```python
from build123d import *

# Parameters (mm, degrees)
F0_R          = 7.6724970278
F1_DEPTH      = 25.4
F1_TAPER      = 3
F1_DEPTH_BACK = 25.4
F1_TAPER_BACK = 3
F4_DEPTH      = 25.4
F4_TAPER      = 3
F4_DEPTH_BACK = 13.716
F6_W          = 8.5597652942
F6_H          = 9.2730754986
F7_DEPTH      = 4.572
F8_R          = 1.5035458926
F9_DEPTH      = 6.5786
F10_R         = 4.568572737
F11_DEPTH     = 53.594


with BuildPart() as f1:
    # F0 (on Front) → F1 (new body, two sides)
    with BuildSketch(Plane.XZ) as f1_sk:
        Circle(F0_R)
    extrude(amount=F1_DEPTH, taper=F1_TAPER)
    extrude(f1_sk.sketch, amount=-F1_DEPTH_BACK, taper=F1_TAPER_BACK)

    # F3 (on offset) → F4 (join, two sides)
    with BuildSketch(Plane.XY.offset(7.366)) as f4_sk:
        Polygon((-3.0564728829, 2.0075347275), (0, -10.3387202816), (3.0564728829, 2.0075347275), (0, 5.0640076103), align=None)
    extrude(amount=F4_DEPTH, taper=F4_TAPER)
    extrude(f4_sk.sketch, amount=-F4_DEPTH_BACK)

    # F6 (on offset) → F7 (join)
    with BuildSketch(Plane.YZ.offset(-6.858)):
        with Locations((-7.6086781919, 0)):
            Rectangle(F6_W, F6_H)
    extrude(amount=-F7_DEPTH)

    # F8 (on face) → F9 (join)
    with BuildSketch(Plane.XZ.offset(11.888560839)):
        with Locations((-9.369360283, 0)):
            Circle(F8_R)
    extrude(amount=F9_DEPTH)

    # F10 (on face) → F11 (cut)
    with BuildSketch(Plane.XZ.offset(25.4)):
        Circle(F10_R)
    extrude(amount=-F11_DEPTH, mode=Mode.SUBTRACT)


solid = f1.part
```
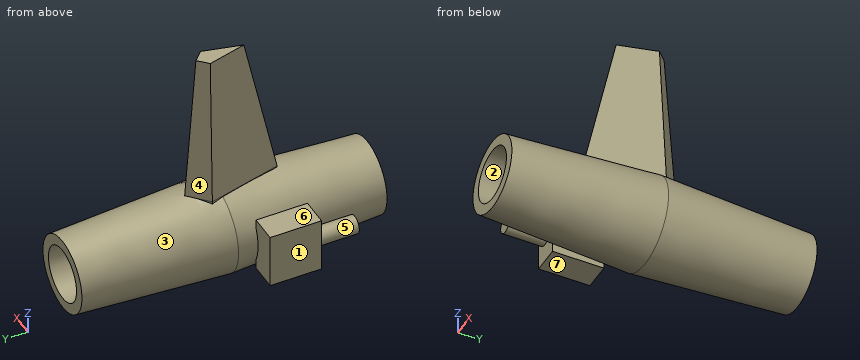
Build history of the part. All positions in model axes, mm. Face numbers are marked on the shaded views. A direction names the side the tool comes from. Round coordinates to 2 decimals unless told otherwise and drop trailing zeros. Loops run counter-clockwise (first coordinate to the right, second up) from the corner with the lowest first, then second, coordinate; pieces in that order, holes last.
Item 1: Two-plate mould, pull along Z, no slides. Class the marked faces 1, 2 and 3: released by +Z, released by -Z, zero draft, split by the parting line, or undercut.
Item 2: Saw through at A-A (z = 22.5). List the corners of the cut face in (x, y), then the cut area to 3 significant figures.
Item 3: Saw through at B-B (y = -20.5). List the corners of the cut face in (x, z), then the cut area to 3 significant figures.
Item 4: Which spindle directions (+Z, -Z, +X, -X, +Y, -Y) get a long thin tool onto all of the face, cutting with end or side? Do the marked faces 4, 5, 6 and 7. Say none if no direction does.
Item 5: Saw through at D-D (z = 27.5). List the corners of the cut face in (x, y).
Item 6: Saw through at C-C (z = 4). State how many separate pieces and enclosed holes the cut face has, then the cut area to 3 significant figures.
Item 7: Pin check, flat tips, straight feed: P1, Ø5, axis at x = -9.5, y = -7.5, coming from the -Z side; P2, Ø5, axis at x = -10, y = -8, coming from the +Z side; P3, Ø4, axis at x = 0, z = -3, coming from the +Y side; P4, Ø1.5, axis at x = -9, z = 0, coming from the -Y side. Stop position of each tip, or through.
Item 8: Drill centre lines: line 1 along Z through (x, y) = (0, -15); line 2 along Y through (x, z) = (-7.5, -2); line 3 along Z through (x, y) = (0, -2). Where is each one in solid material? Low to high.
Worked answers:
1. face 1: zero draft
1. face 2: undercut
1. face 3: split by the parting line
2. outline: (-2.18, 1.76) - (0, -7.04) - (2.18, 1.76) - (0, 3.94) - close
2. area: 23.9 mm2
3. outline: circle Ø13.2 at (0, 0); hole circle Ø9.14 at (0, 0)
3. area: 71.2 mm2
4. face 4: +Z, -X, +Y
4. face 5: -Y
4. face 6: +Z, -X, +Y, -Y
4. face 7: -Z, -X, +Y, -Y
5. outline: (-1.89, 1.68) - (0, -5.95) - (1.89, 1.68) - (0, 3.57) - close
6. separate pieces: 3
6. enclosed holes: 0
6. area: 399 mm2
7. P1: stops at z = -4.64
7. P2: stops at z = 4.64
7. P3: stops at y = 25.4
7. P4: stops at y = -18.47
8. line 1: z = -6.89 to -4.57, 4.57 to 6.89
8. line 2: y = -11.89 to -3.33
8. line 3: z = -7.57 to -4.57, 4.57 to 32.77
